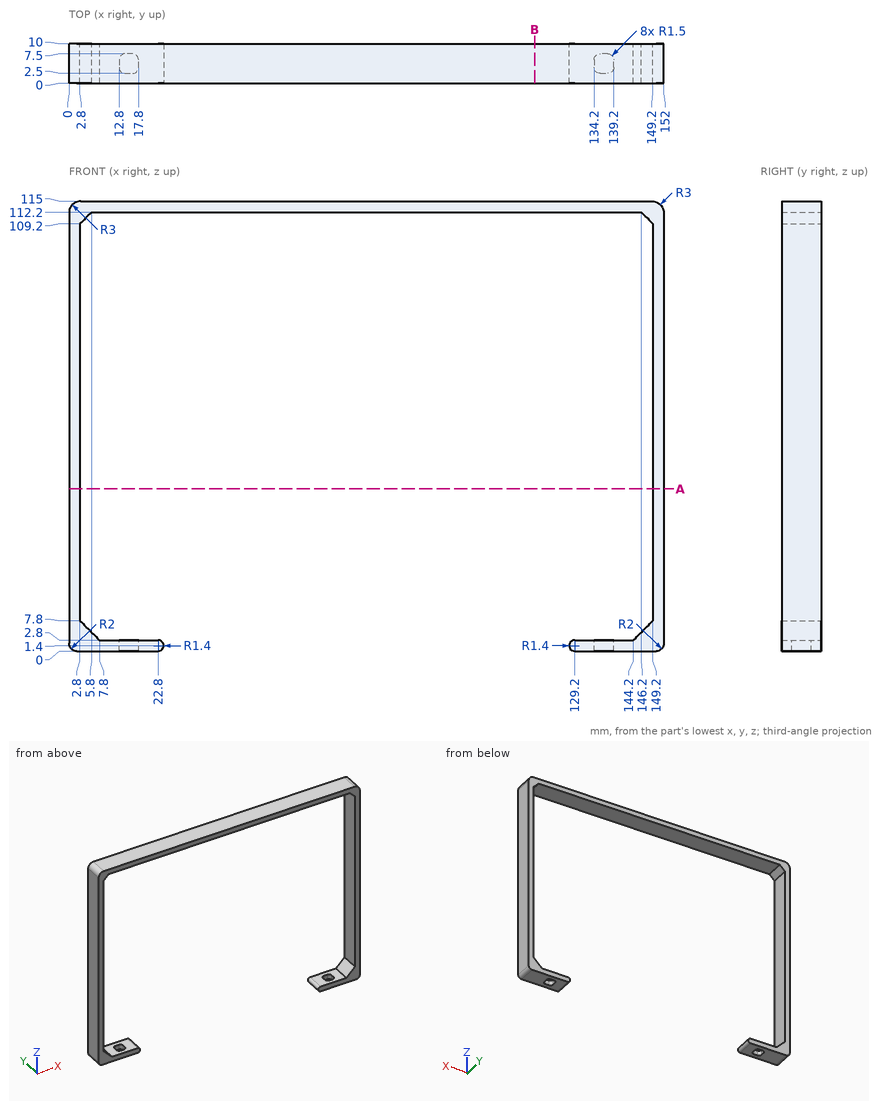
Check sheet for the drawn part. Datum: minimum x, y, z corner. Units: mm. Round coordinates to 2 decimals unless told otherwise and drop trailing zeros. Loops run counter-clockwise (first coordinate to the right, second up) from the corner with the lowest first, then second, coordinate; pieces in that order, holes last. Notation, with made-up numbers: (-31.75, 64.5) - (-6.75, 64.5) arc R35 ccw to (-6.75, 96.5) - close; hole circle Ø10 at (52, 53). An arc over 180 degrees is marked (long way). Write item = value, one per line. Start each with the question number.
1. Depth check by flat-ended pin: pin 1 (1 mm diameter, centred on y = 5.5, z = 1, fed in from +X); pin 2 (5 mm diameter, centred on x = 65.5, y = 7, fed in from -Z); pin 3 (0.6 mm diameter, centred on y = 5.5, z = 1, fed in from -X). Enter the tip coordinate at first touch or a pass-through.
2. Section check A-A on z = 41.5. Enter the section's corners in (x, y).
3. Section check B-B on x = 119. Enter the section's corners in (y, z).
4. Thickness scan on line 1 (X direction, y = 5, z = 74.5); line 2 (Z direction, x = 11.5, y = 6.25); line 3 (Z direction, x = 114, y = 2.75). Record the ranges inside material, lowest first.
Working result:
q1.pin_1 = 151.94
q1.pin_2 = 112.2
q1.pin_3 = 0.13
q2.outline = (0, 0) - (2.8, 0) - (2.8, 10) - (0, 10) - close; (149.2, 0) - (152, 0) - (152, 10) - (149.2, 10) - close
q3.outline = (0, 112.2) - (10, 112.2) - (10, 115) - (0, 115) - close
q4.line_1 = 0 to 2.8, 149.2 to 152
q4.line_2 = 0 to 2.8, 112.2 to 115
q4.line_3 = 112.2 to 115
